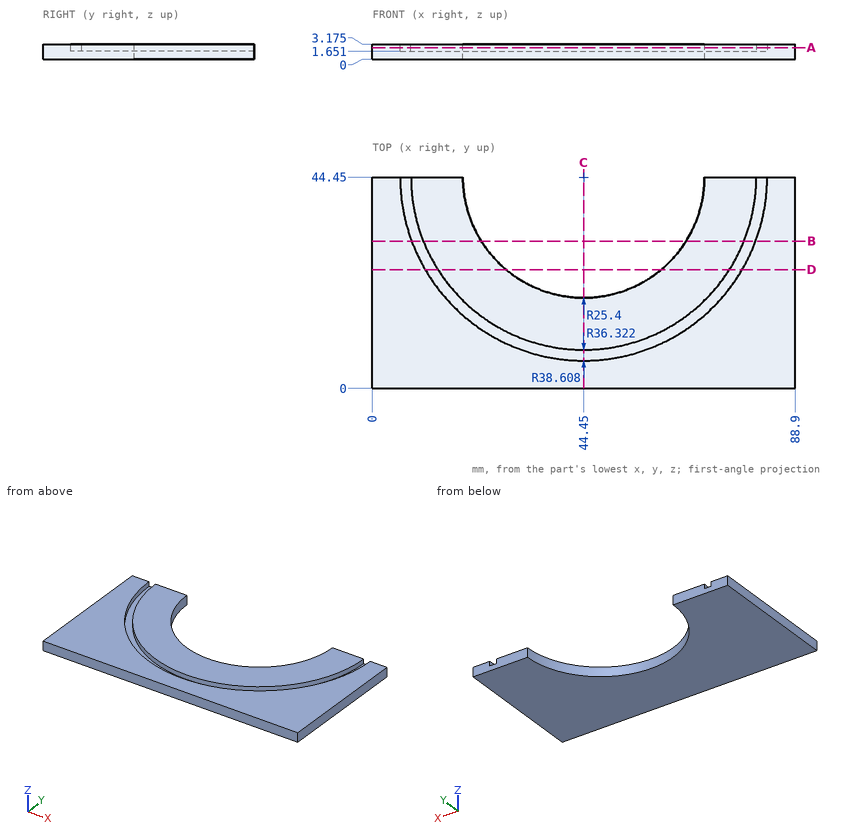
Check sheet for the drawn part. Datum: minimum x, y, z corner. Units: mm. Round coordinates to 2 decimals unless told otherwise and drop trailing zeros. Order: outer loops, then holes, each group sorted by start corner. A loop starts at its lowest first (then second) coordinate and runs counter-clockwise, first axis right, second up. Notation, with made-up numbers: (81, 55.25) -> (93, 55.25) arc R17 cw to (93, 84.25) -> close; hole circle Ø10 at (-20, -38). An arc over 180 degrees is marked (long way). Put each result on its own line as item: value. Start each with the question number.
(1) Section check D-D (y = 25). Enter the section's corners in (x, z) (3 decimals).
(2) Section check B-B (y = 31). Enter the section's corners in (x, z) (3 decimals).
(3) Material ranges on line 1 along X through (y, z) = (26.5, 2.15); line 2 along Z through (x, y) = (66, 15); line 3 along X through (y, z) = (25.5, 1.3), recorded low to high.
(4) Section check C-C (x = 44.45). Enter the section's corners in (y, z) (3 decimals).
(5) Section check A-A (z = 2.4). Enter the section's corners in (x, y), then the cut area to 3 significant figures.
Completed:
1. outline: (0, 0) -> (28.114, 0) -> (28.114, 3.175) -> (13.775, 3.175) -> (13.775, 1.651) -> (11.099, 1.651) -> (11.099, 3.175) -> (0, 3.175) -> close; (60.786, 0) -> (88.9, 0) -> (88.9, 3.175) -> (77.801, 3.175) -> (77.801, 1.651) -> (75.125, 1.651) -> (75.125, 3.175) -> (60.786, 3.175) -> close
2. outline: (0, 0) -> (22.903, 0) -> (22.903, 3.175) -> (10.71, 3.175) -> (10.71, 1.651) -> (8.261, 1.651) -> (8.261, 3.175) -> (0, 3.175) -> close; (65.997, 0) -> (88.9, 0) -> (88.9, 3.175) -> (80.639, 3.175) -> (80.639, 1.651) -> (78.19, 1.651) -> (78.19, 3.175) -> (65.997, 3.175) -> close
3. line 1: x = 0 to 10.27, 12.87 to 26.48, 62.42 to 76.03, 78.63 to 88.9
3. line 2: z = 0 to 1.65
3. line 3: x = 0 to 27.54, 61.36 to 88.9
4. outline: (0, 0) -> (19.05, 0) -> (19.05, 3.175) -> (8.128, 3.175) -> (8.128, 1.651) -> (5.842, 1.651) -> (5.842, 3.175) -> (0, 3.175) -> close
5. outline: (0, 0) -> (88.9, 0) -> (88.9, 44.45) -> (83.06, 44.45) arc R38.61 cw to (5.84, 44.45) -> (0, 44.45) -> close; (8.13, 44.45) arc R36.32 ccw to (80.77, 44.45) -> (69.85, 44.45) arc R25.4 cw to (19.05, 44.45) -> close
5. area: 2,670 mm2
